```python
from build123d import *

# Parameters (mm, degrees)
SKETCH_1_R          = 37
SKETCH_1_R_2        = 2.5
SKETCH_1_R_3        = 17
EXTRUDE_1_DEPTH     = 7
SKETCH_4_R          = 7.5
EXTRUDE_9_DEPTH     = 10
CUT_EXTRUDE_1_REACH = 57.018
SKETCH_2_R          = 3.1
CHAMFER_1_SIZE      = 1


with BuildPart() as part:
    # 草图1 → 凸台-拉伸1 (new body)
    with BuildSketch(Plane(origin=(0, 0, 0), x_dir=(1, 0, 0), z_dir=(0, 1, 0))):
        with Locations(Location((0, 0, 0), (0, 0, 270))):
            Circle(SKETCH_1_R)
        with Locations(Location((21, 0, 0), (0, 0, 270))):
            Circle(SKETCH_1_R_2, mode=Mode.SUBTRACT)
        with Locations(Location((0, -21, 0), (0, 0, 270))):
            Circle(SKETCH_1_R_2, mode=Mode.SUBTRACT)
        with Locations(Location((-21, 0, 0), (0, 0, 270))):
            Circle(SKETCH_1_R_2, mode=Mode.SUBTRACT)
        with Locations(Location((0, 21, 0), (0, 0, 270))):
            Circle(SKETCH_1_R_2, mode=Mode.SUBTRACT)
        with Locations(Location((0, 0, 0), (0, 0, 270))):
            Circle(SKETCH_1_R_3, mode=Mode.SUBTRACT)
    extrude(amount=EXTRUDE_1_DEPTH)

    # 草图4 → 凸台-拉伸9 (add)
    with BuildSketch(Plane(origin=(0, 7, 0), x_dir=(1, 0, 0), z_dir=(0, 1, 0))):
        with Locations(Location((20.859650045, -20.859650045, 0), (0, 0, 314.999668768))):
            Circle(SKETCH_4_R)
        with Locations(Location((-20.859650045, -20.859650045, 0), (0, 0, 224.999668649))):
            Circle(SKETCH_4_R)
        with Locations(Location((-20.859650045, 20.859650045, 0), (0, 0, 134.999668649))):
            Circle(SKETCH_4_R)
        with Locations(Location((20.859650045, 20.859650045, 0), (0, 0, 44.999668649))):
            Circle(SKETCH_4_R)
    extrude(amount=EXTRUDE_9_DEPTH)

    # 草图2 → 切除-拉伸1 (cut, up to next)
    with BuildSketch(Plane.XZ, mode=Mode.PRIVATE) as cut_extrude_1_sk1:
        with Locations(Location((20.859650045, 20.859650045, 0), (0, 0, 270))):
            Circle(SKETCH_2_R)
    cut_extrude_1_tool1 = extrude(cut_extrude_1_sk1.sketch, amount=-CUT_EXTRUDE_1_REACH, mode=Mode.PRIVATE) & part.part
    # 草图2 → 切除-拉伸1 (cut, up to next)
    with BuildSketch(Plane.XZ, mode=Mode.PRIVATE) as cut_extrude_1_sk2:
        with Locations(Location((20.859650045, -20.859650045, 0), (0, 0, 270))):
            Circle(SKETCH_2_R)
    cut_extrude_1_tool2 = extrude(cut_extrude_1_sk2.sketch, amount=-CUT_EXTRUDE_1_REACH, mode=Mode.PRIVATE) & part.part
    # 草图2 → 切除-拉伸1 (cut, up to next)
    with BuildSketch(Plane.XZ, mode=Mode.PRIVATE) as cut_extrude_1_sk3:
        with Locations(Location((-20.859650045, -20.859650045, 0), (0, 0, 270))):
            Circle(SKETCH_2_R)
    cut_extrude_1_tool3 = extrude(cut_extrude_1_sk3.sketch, amount=-CUT_EXTRUDE_1_REACH, mode=Mode.PRIVATE) & part.part
    # 草图2 → 切除-拉伸1 (cut, up to next)
    with BuildSketch(Plane.XZ, mode=Mode.PRIVATE) as cut_extrude_1_sk4:
        with Locations(Location((-20.859650045, 20.859650045, 0), (0, 0, 270))):
            Circle(SKETCH_2_R)
    cut_extrude_1_tool4 = extrude(cut_extrude_1_sk4.sketch, amount=-CUT_EXTRUDE_1_REACH, mode=Mode.PRIVATE) & part.part
    add(cut_extrude_1_tool1.solids().sort_by_distance((20.85965, 0, 20.85965))[0], mode=Mode.SUBTRACT)
    add(cut_extrude_1_tool2.solids().sort_by_distance((20.85965, 0, -20.85965))[0], mode=Mode.SUBTRACT)
    add(cut_extrude_1_tool3.solids().sort_by_distance((-20.85965, 0, -20.85965))[0], mode=Mode.SUBTRACT)
    add(cut_extrude_1_tool4.solids().sort_by_distance((-20.85965, 0, 20.85965))[0], mode=Mode.SUBTRACT)

    # 倒角1
    chamfer_1_edges = [part.edges().sort_by_distance(p)[0] for p in [
        (15.556379845, 17, 15.556318527),
        (-15.556318516, 17, 15.556379856),
        (-15.556379856, 17, -15.556318516),
        (15.556318516, 17, -15.556379856),
        (-20.859650045, 17, 23.959650045),
        (-20.859650045, 0, 23.959650045),
        (-20.859650045, 17, -17.759650045),
        (-20.859650045, 0, -17.759650045),
        (20.859650045, 17, -17.759650045),
        (20.859650045, 0, -17.759650045),
        (20.859650045, 17, 23.959650045),
        (20.859650045, 0, 23.959650045),
    ]]
    chamfer(chamfer_1_edges, length=CHAMFER_1_SIZE)


solid = part.part
```
Verification items for the finished model (mm, model axes). A direction names the side the tool comes from. Coordinates: 2 decimals unless noted, no trailing zeros. Loops run counter-clockwise (first coordinate to the right, second up) from the corner with the lowest first, then second, coordinate; pieces in that order, holes last. Notation, with made-up numbers: (81.5, 73.5) -> (96.5, 73.5) arc R11 cw to (96.5, 89.5) -> close; hole circle Ø4 at (35.25, 26.25). An arc over 180 degrees is marked (long way). Put each result on its own line as item: value.
1. Section check A-A, the plane x = 0. Record the boundary of the cut face in (y, z), then the cut area to 3 significant figures.
Result set:
outline: (0, -37) -> (7, -37) -> (7, -23.5) -> (0, -23.5) -> close; (0, -18.5) -> (7, -18.5) -> (7, -17) -> (0, -17) -> close; (0, 17) -> (7, 17) -> (7, 18.5) -> (0, 18.5) -> close; (0, 23.5) -> (7, 23.5) -> (7, 37) -> (0, 37) -> close
area: 210 mm^2
2. Tool access check on faces 1 (the face through (24, 17, 24)), 2 (the face through (-15.33, 11.44, 15.79)). Record the directions out of +Z, -Z, +X, -X, +Y, -Y that give a thin tool (end or side, any length) a straight path to the whole face; none if there is none.
Result set:
face 1: +Z, -Z, +X, -X, +Y
face 2: +Y
3. Section check C-C, the plane z = -7. Record the boundary of the cut face in (x, y), then the cut area to 3 significant figures.
Result set:
outline: (-36.33, 0) -> (-15.49, 0) -> (-15.49, 7) -> (-36.33, 7) -> close; (15.49, 0) -> (36.33, 0) -> (36.33, 7) -> (15.49, 7) -> close
area: 292 mm^2
4. Thickness scan on line 1 (X direction, y = 5.5, z = 21); line 2 (Y direction, x = -3, z = -29); line 3 (X direction, y = 3.75, z = 19). Record the ranges inside material, lowest first.
Result set:
line 1: x = -30.46 to -23.96, -17.76 to -2.5, 2.5 to 17.76, 23.96 to 30.46
line 2: y = 0 to 7
line 3: x = -31.75 to -23.34, -18.38 to -1.5, 1.5 to 18.38, 23.34 to 31.75
5. Gauge pin test, flat ends, axial feed: P1, Ø8, axis at x = 13, y = 3.5, coming from the +Z side; P2, Ø6, axis at x = 23, y = 5.5, coming from the -Z side; P3, Ø8, axis at x = 20.86, z = 20.86, coming from the +Y side. Record the tip position at first contact, or that the pin passes through.
Result set:
P1: stops at z = 35.89
P2: stops at z = -31.13
P3: stops at y = 16.9
6. Section check D-D, the plane x = 11. Record the boundary of the cut face in (y, z), then the cut area to 3 significant figures.
Result set:
outline: (0, -35.33) -> (7, -35.33) -> (7, -12.96) -> (0, -12.96) -> close; (0, 12.96) -> (7, 12.96) -> (7, 35.33) -> (0, 35.33) -> close
area: 313 mm^2
7. Mould release check, pull along Z, two halves, no side actions. Record for faces 3 (the face through (-8, 0, 16)), 4 (the face through (-18.25, 8.4, -22.53)): pulls with the +Z half, pulls with the -Z half, needs draft (parallel to the pull), parting line crosses it, or undercut.
Result set:
face 3: needs draft
face 4: undercut
8. Section check B-B, the plane y = 8.5. Record the boundary of the cut face in (x, z).
Result set:
outline: circle Ø15 at (-20.86, -20.86); circle Ø15 at (-20.86, 20.86); circle Ø15 at (20.86, -20.86); circle Ø15 at (20.86, 20.86); hole circle Ø6.2 at (-20.86, -20.86); hole circle Ø6.2 at (-20.86, 20.86); hole circle Ø6.2 at (20.86, -20.86); hole circle Ø6.2 at (20.86, 20.86)
